The model under review builds one solid part; all positions refer to its coordinate system, in mm. A direction names the side the tool comes from. Coordinates: 2 decimals unless noted, no trailing zeros. Loops run counter-clockwise (first coordinate to the right, second up) from the corner with the lowest first, then second, coordinate; pieces in that order, holes last. Notation, with made-up numbers: M 35,7 L 47,7 A19 cw 47,27 Z; hole C 6,-5.5 d9. An arc over 180 degrees is marked long. Return JSON: item names as keys, results as strings.
```python
from build123d import *
from OCP.BRepFilletAPI import BRepFilletAPI_MakeChamfer

# Parameters (mm, degrees)
SKETCH1_W           = 140.96
SKETCH1_H           = 6.3
BOSS_EXTRUDE1_DEPTH = 6
SKETCH2_W           = 6.5
SKETCH2_H           = 6.3
BOSS_EXTRUDE2_DEPTH = 8
SKETCH3_W           = 71.75
SKETCH3_H           = 1.57
SKETCH3_W_2         = 60.6
CUT_EXTRUDE1_DEPTH  = 13
CHAMFER1_SIZE       = 0.5
SKETCH5_W           = 8.468797777
SKETCH5_H           = 7.958933252
SKETCH5_W_2         = 8.892237666
BOSS_EXTRUDE3_DEPTH = 4
CHAMFER2_SIZE       = 2
CHAMFER2_SIZE2      = 8


with BuildPart() as part:
    # Sketch1 → Boss-Extrude1 (new body)
    with BuildSketch(Plane(origin=(0, 0, 0), x_dir=(1, 0, 0), z_dir=(0, 1, 0))):
        Rectangle(SKETCH1_W, SKETCH1_H)
    extrude(amount=BOSS_EXTRUDE1_DEPTH)

    # Sketch2 → Boss-Extrude2 (add)
    with BuildSketch(Plane(origin=(0, 6, 0), x_dir=(1, 0, 0), z_dir=(0, 1, 0))):
        with Locations((67.23, 0)):
            Rectangle(SKETCH2_W, SKETCH2_H)
        with Locations((-67.23, 0)):
            Rectangle(SKETCH2_W, SKETCH2_H)
    extrude(amount=BOSS_EXTRUDE2_DEPTH)

    # Sketch3 → Cut-Extrude1 (cut)
    with BuildSketch(Plane(origin=(0, 14, 0), x_dir=(1, 0, 0), z_dir=(0, 1, 0))):
        with Locations((-30.995, 0)):
            Rectangle(SKETCH3_W, SKETCH3_H)
        with Locations((36.57, 0)):
            Rectangle(SKETCH3_W_2, SKETCH3_H)
    extrude(amount=-CUT_EXTRUDE1_DEPTH, mode=Mode.SUBTRACT)

    # Chamfer1
    chamfer1_edges = [part.edges().sort_by_distance(p)[0] for p in [
        (-65.425, 14, -0.785),
        (65.425, 14, 0.785),
        (-65.425, 14, 0.785),
        (-66.87, 14, 0),
        (-29.55, 6, -0.785),
        (-29.55, 6, 0.785),
        (66.87, 14, 0),
        (65.425, 14, -0.785),
        (35.125, 6, 0.785),
        (35.125, 6, -0.785),
    ]]
    chamfer(chamfer1_edges, length=CHAMFER1_SIZE)

    # Sketch5 → Boss-Extrude3 (add)
    with BuildSketch(Plane(origin=(0, 14, 0), x_dir=(1, 0, 0), z_dir=(0, 1, 0))):
        with Locations((-68.255348276, 0)):
            Rectangle(SKETCH5_W, SKETCH5_H)
        with Locations((68.374589196, 0)):
            Rectangle(SKETCH5_W_2, SKETCH5_H)
    extrude(amount=BOSS_EXTRUDE3_DEPTH)

    # Chamfer2: one chamfer whose edges measure the first distance from different faces: ONE call of the kernel's chamfer builder (chamfer() names one face for all edges)
    chamfer2_edges_1 = [part.edges().sort_by_distance(p)[0] for p in [
        (-64.020949387, 18, 0),
    ]]
    chamfer2_side_1 = [part.faces().sort_by_distance(p)[0] for p in [
        (-64.020949387, 16, 0),
    ]]
    chamfer2_edges_2 = [part.edges().sort_by_distance(p)[0] for p in [
        (63.928470363, 18, 0),
    ]]
    chamfer2_side_2 = [part.faces().sort_by_distance(p)[0] for p in [
        (63.928470363, 16, 0),
    ]]
    chamfer2 = BRepFilletAPI_MakeChamfer(part.part.solid().wrapped)
    for e in chamfer2_edges_1:
        chamfer2.Add(CHAMFER2_SIZE, CHAMFER2_SIZE2, e.wrapped, chamfer2_side_1[0].wrapped)  # the first distance lies on this face
    for e in chamfer2_edges_2:
        chamfer2.Add(CHAMFER2_SIZE, CHAMFER2_SIZE2, e.wrapped, chamfer2_side_2[0].wrapped)  # the first distance lies on this face
    add(Compound.cast(chamfer2.Shape()), mode=Mode.REPLACE)


solid = part.part
```
1. The part is to be moulded in two halves that separate along Z. For faces 5 (the face through (-34, 3, -0.785)), 6 (the face through (-1, 2, -3.15)), 7 (the face through (-68.077, 17.014, 0.056)), say which applies: released by +Z, released by -Z, zero draft, split by the parting line, or undercut.
Check values:
{"face 5": "undercut", "face 6": "released by -Z", "face 7": "zero draft"}
2. Insertion check: pin 1 Ø1.2 at (y, z) = (9.5, -2) entering from +X; pin 2 Ø0.5 at (x, z) = (46, 0) entering from +Y; pin 3 Ø3 at (y, z) = (6.5, 1) entering from -X. Each pin has a flat end and moves straight along its axis. Give the tip position at first contact, or say it passes through.
Check values:
{"pin 1": "x = 70.48", "pin 2": "y = 1", "pin 3": "x = -70.48"}
3. Add section A-A on y = 3.25. Give the boundary of the cut face in (x, z) (3 decimals).
Check values:
{"outline": "M -70.48,-3.15 L 70.48,-3.15 L 70.48,3.15 L -70.48,3.15 Z; hole M -66.87,-0.785 L 4.88,-0.785 L 4.88,0.785 L -66.87,0.785 Z; hole M 6.27,-0.785 L 66.87,-0.785 L 66.87,0.785 L 6.27,0.785 Z"}
4. Add section B-B on y = 11.5. Give the boundary of the cut face in (x, z) (3 decimals), plus the area to 3 significant figures.
Check values:
{"outline": "M -70.48,-3.15 L -63.98,-3.15 L -63.98,-0.785 L -66.87,-0.785 L -66.87,0.785 L -63.98,0.785 L -63.98,3.15 L -70.48,3.15 Z; M 63.98,-3.15 L 70.48,-3.15 L 70.48,3.15 L 63.98,3.15 L 63.98,0.785 L 66.87,0.785 L 66.87,-0.785 L 63.98,-0.785 Z", "area": "72.8 mm²"}
5. Add section C-C on x = -12. Give the boundary of the cut face in (y, z) (3 decimals).
Check values:
{"outline": "M 0,-3.15 L 6,-3.15 L 6,-1.285 L 5.5,-0.785 L 1,-0.785 L 1,0.785 L 5.5,0.785 L 6,1.285 L 6,3.15 L 0,3.15 Z"}
6. To check wall thickness, follow line 1 (X direction, y = 5.75, z = 0); line 2 (X direction, y = 10, z = -2); line 3 (X direction, y = 14.5, z = 1.25). State the ranges of each line that lie inside material, in increasing order.
Check values:
{"line 1": "-70.48 to -66.87, 4.88 to 6.27, 66.87 to 70.48", "line 2": "-70.48 to -63.98, 63.98 to 70.48", "line 3": "-72.49 to -64.02, 63.93 to 72.82"}
7. Machinability: for faces 1 (the face through (-1, 0, 0)), 2 (the face through (6.27, 4, 0)), 3 (the face through (70.48, 7, 0)), 4 (the face through (-66, 14, 0)), which of the approach directions +Z, -Z, +X, -X, +Y, -Y give a long, thin tool a straight path to every point of the face, cutting with its end or side? Answer none if there is none.
Check values:
{"face 1": "+Z, -Z, +X, -X, -Y", "face 2": "+Y", "face 3": "+Z, -Z, +X, -Y", "face 4": "none"}
